from build123d import *

# Parameters (mm, degrees)
SKETCH1_W           = 172.72
SKETCH1_H           = 38.1
BOSS_EXTRUDE1_DEPTH = 7
SKETCH2_R           = 1.778
CUT_EXTRUDE1_DEPTH  = 17
SKETCH3_W           = 20
SKETCH3_H           = 8
BOSS_EXTRUDE2_DEPTH = 12
SKETCH4_R           = 0.5
CUT_EXTRUDE2_DEPTH  = 10
CHAMFER1_SIZE       = 12
CHAMFER2_SIZE       = 2
CHAMFER3_SIZE       = 5


# Some blends are built 0.0001 mm under size
with BuildPart() as part:
    # Sketch1 → Boss-Extrude1 (new body)
    with BuildSketch(Plane(origin=(0, 0, 0), x_dir=(1, 0, 0), z_dir=(0, 1, 0))):
        with Locations((7.116134283, -6.04768057)):
            Rectangle(SKETCH1_W, SKETCH1_H)
    extrude(amount=BOSS_EXTRUDE1_DEPTH)

    # Sketch2 → Cut-Extrude1 (cut)
    with BuildSketch(Plane(origin=(0, 7, 0), x_dir=(1, 0, 0), z_dir=(0, 1, 0))):
        with Locations(Location((-69.083865717, 6.65231943, 0), (0, 0, 270))):
            Circle(SKETCH2_R)
        with Locations(Location((-69.083865717, -18.74768057, 0), (0, 0, 270))):
            Circle(SKETCH2_R)
        with Locations(Location((83.316134283, 6.65231943, 0), (0, 0, 270))):
            Circle(SKETCH2_R)
        with Locations(Location((83.316134283, -18.74768057, 0), (0, 0, 270))):
            Circle(SKETCH2_R)
    extrude(amount=-CUT_EXTRUDE1_DEPTH, mode=Mode.SUBTRACT)

    # Sketch3 → Boss-Extrude2 (add)
    with BuildSketch(Plane(origin=(0, 7, 0), x_dir=(1, 0, 0), z_dir=(0, 1, 0))):
        with Locations((-4.723865717, 6.00231943)):
            Rectangle(SKETCH3_W, SKETCH3_H)
        with Locations((39.276134283, 6.00231943)):
            Rectangle(SKETCH3_W, SKETCH3_H)
    extrude(amount=BOSS_EXTRUDE2_DEPTH)

    # Sketch4 → Cut-Extrude2 (cut)
    with BuildSketch(Plane(origin=(0, 0, -10.00231943), x_dir=(-1, 0, 0), z_dir=(0, 0, -1))):
        with Locations((-31.776134283, 16.85)):
            Circle(SKETCH4_R)
        with Locations((-31.776134283, 9.35)):
            Circle(SKETCH4_R)
        with Locations((-2.776134283, 9.35)):
            Circle(SKETCH4_R)
        with Locations((-2.776134283, 16.85)):
            Circle(SKETCH4_R)
    extrude(amount=-CUT_EXTRUDE2_DEPTH, mode=Mode.SUBTRACT)

    # Chamfer1
    chamfer1_edges = [part.edges().sort_by_distance(p)[0] for p in [
        (49.276134283, 7, -6.00231943),
        (-14.723865717, 7, -6.00231943),
    ]]
    chamfer(chamfer1_edges, length=CHAMFER1_SIZE - 0.0001)  # a hair under: the kernel refuses the full size

    # Chamfer2
    chamfer2_edges = [part.edges().sort_by_distance(p)[0] for p in [
        (93.476134283, 7, 6.04768057),
        (-79.243865717, 7, 6.04768057),
        (7.116134283, 7, 25.09768057),
    ]]
    chamfer(chamfer2_edges, length=CHAMFER2_SIZE)

    # Chamfer3
    # the kernel refuses this chamfer: 5 mm, written as the material it takes off along each edge
    with BuildSketch(Plane(origin=(93.476134283, -12.85841494, -13.00231943), x_dir=(-0.9996219169112968, 0, -0.027495876610586282), z_dir=(0, 1, 0)), Plane(origin=(93.476134283, -12.85841494, 25.09768057), x_dir=(0.0274958766105877, 0, -0.9996219169112968), z_dir=(0, 1, 0))) as chamfer3_piece_1:
        Polygon((CHAMFER3_SIZE * 0.999621916911, CHAMFER3_SIZE * 0.0274958766106), (-CHAMFER3_SIZE * 0.0274958766106, CHAMFER3_SIZE * 0.999621916911), (0, 0), align=None)
    extrude(amount=30.71682988, mode=Mode.SUBTRACT)
    with BuildSketch(Plane(origin=(-79.243865717, -12.85841494, 25.09768057), x_dir=(-0.0274958766105877, 0, -0.9996219169112968), z_dir=(0, 1, 0)), Plane(origin=(-79.243865717, -12.85841494, -13.00231943), x_dir=(0.9996219169112968, 0, -0.027495876610586282), z_dir=(0, 1, 0))) as chamfer3_piece_2:
        Polygon((CHAMFER3_SIZE * 0.999621916911, -CHAMFER3_SIZE * 0.0274958766106), (-CHAMFER3_SIZE * 0.0274958766106, -CHAMFER3_SIZE * 0.999621916911), (0, 0), align=None)
    extrude(amount=30.71682988, mode=Mode.SUBTRACT)


solid = part.part
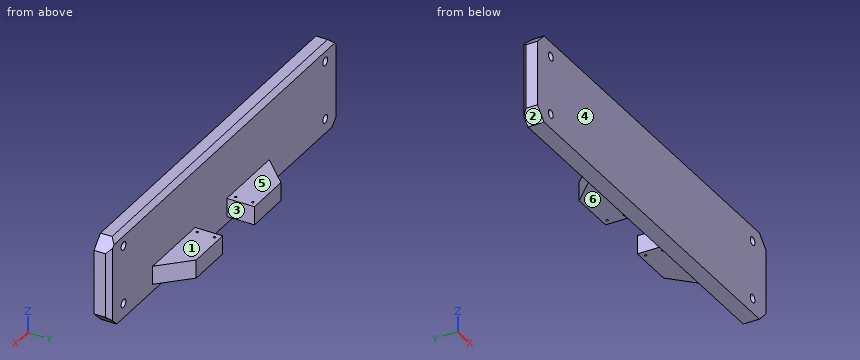
Source: CAD feature listing. Evaluate the final solid. Frame: model axes, mm. Face numbers are marked on the shaded views. A direction names the side the tool comes from. Round coordinates to 2 decimals unless told otherwise and drop trailing zeros. Loops run counter-clockwise (first coordinate to the right, second up) from the corner with the lowest first, then second, coordinate; pieces in that order, holes last.
Q1. First-contact query: P1, Ø9.5, axis at x = -16.5, y = 15.5, coming from the +Z side; P2, Ø4.5, axis at x = 83.32, z = 18.75, coming from the +Y side; P3, Ø1, axis at x = 0.5, y = 11, coming from the -Z side; P4, Ø6, axis at x = 23, y = 12, coming from the +Z side. Flat tips, straight axial feed; report the tip coordinate or a pass-through.
Q2. Access query for the marked faces 4, 5 and 6. Directions: +Z, -Z, +X, -X, +Y, -Y. A direction counts if a zero-diameter tool reaches every point of the face in a straight line with its end or side. Return the directions, or none.
Q3. Section B-B, the plane x = 63. Return loops of the section in (y, z).
Q4. Section C-C, the plane z = 2. Return loops of the section in (x, y).
Q5. Section D-D, the plane x = -20. Return loops of the section in (y, z), plus the area to 3 significant figures.
Q6. Ray query, line 1 (Z direction, x = -5, y = 12); line 2 (Y direction, x = 18.5, z = -8); line 3 (X direction, y = 11, z = -5). Return the intervals inside material, ascending.
Q7. Section A-A, the plane y = 12.75. Return loops of the section in (x, z).
Q8. Mould query, pull axis X, two halves, no side actions, for the marked faces 1, 2 and 3. Classes: pulls with the +X half, pulls with the -X half, needs draft (parallel to the pull), parting line crosses it, or undercut.
Solutions:
1. P1: stops at z = -2
1. P2: stops at y = 7
1. P3: stops at z = -10
1. P4: passes through
2. face 4: +Z, -Z, +X, -X, -Y
2. face 5: +Z, +X, -X, +Y
2. face 6: -Z, +X, -X, +Y
3. outline: (0, -13) - (7, -13) - (7, 23.1) - (5, 25.1) - (0, 25.1) - close
4. outline: (-79.24, 0) - (93.48, 0) - (93.48, 5) - (91.48, 7) - (-77.24, 7) - (-79.24, 5) - close
5. outline: (0, -13) - (7, -13) - (7, -10) - (13.72, -10) - (13.72, -2) - (7, -2) - (7, 23.1) - (5, 25.1) - (0, 25.1) - close
5. area: 318 mm2
6. line 1: z = -10 to -2
6. line 2: y = 0 to 7
6. line 3: x = -22.72 to 5.28, 29.28 to 57.28
7. outline: (-20.97, -10) - (5.28, -10) - (5.28, -2) - (-20.97, -2) - close; (29.28, -10) - (55.53, -10) - (55.53, -2) - (29.28, -2) - close
8. face 1: needs draft
8. face 2: pulls with the -X half
8. face 3: undercut
